Could you check a few things on this drawing? It's one solid part, dimensions in mm from its lowest x, y, z. Round coordinates to 2 decimals unless told otherwise and drop trailing zeros. Loops run counter-clockwise (first coordinate to the right, second up) from the corner with the lowest first, then second, coordinate; pieces in that order, holes last. Notation, with made-up numbers: M 30,64.25 L 83,64.25 A19 cw 83,92.25 Z; hole C 56.5,-2.5 d8. An arc over 180 degrees is marked long. Return JSON: item names as keys, results as strings.
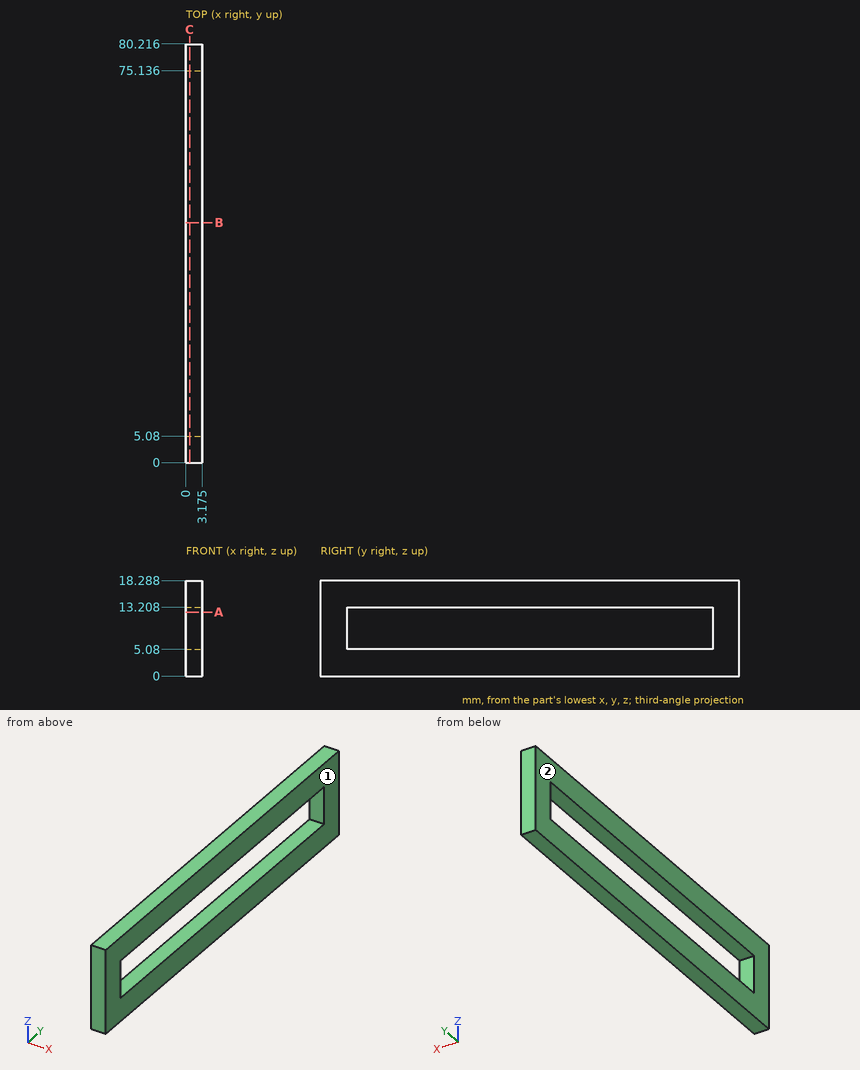
Q1. Suppose I cut it at A-A, the plane z = 12.25. Please give me the cut outline in (x, y) (1 decimal).
Results:
{"outline": "M 0,0 L 3.2,0 L 3.2,5.1 L 0,5.1 Z; M 0,75.1 L 3.2,75.1 L 3.2,80.2 L 0,80.2 Z"}
Q2. I'm going to push flat-ended pins straight in: pin 1 Ø1.5 at (y, z) = (22, 11.5) entering from +X; pin 2 Ø2 at (y, z) = (64, 13.5) entering from -X. Where does each tip first touch, or does it pass through?
Results:
{"pin 1": "passes through", "pin 2": "stops at x = 0"}
Q3. Suppose I cut it at B-B, the plane y = 46. Please give me the cut outline in (x, z) (3 decimals).
Results:
{"outline": "M 0,0 L 3.175,0 L 3.175,5.08 L 0,5.08 Z; M 0,13.208 L 3.175,13.208 L 3.175,18.288 L 0,18.288 Z"}
Q4. If I drill on line 1 along Y through (x, z) = (2.15, 12); line 2 along Z through (x, y) = (1.3, 64.5), over which ranges is the centre line in solid material (lowest first)?
Results:
{"line 1": "y = 0 to 5.08, 75.14 to 80.22", "line 2": "z = 0 to 5.08, 13.21 to 18.29"}
Q5. Thinking about a two-plate mould opening in X: for the marked faces 1 and 2, which applies, pulls with the +X half, pulls with the -X half, needs draft (parallel to the pull), parting line crosses it, or undercut?
Results:
{"face 1": "pulls with the +X half", "face 2": "pulls with the -X half"}
Q6. Suppose I cut it at C-C, the plane x = 0.7. Please give me the cut outline in (y, z).
Results:
{"outline": "M 0,0 L 80.22,0 L 80.22,18.29 L 0,18.29 Z; hole M 5.08,5.08 L 75.14,5.08 L 75.14,13.21 L 5.08,13.21 Z"}
